Model file for the job. Use its own axes, mm. A direction names the side the tool comes from. Coordinates: 2 decimals unless noted, no trailing zeros. Write each loop counter-clockwise with the first axis right and the second up, starting at its lowest first coordinate (ties: lowest second). Pieces come first, ordered by that corner, then holes. Notation, with made-up numbers: M -23.75,89.5 L -5.75,89.5 A18 cw -5.75,101.5 Z; hole C -23,-14.5 d7. An arc over 180 degrees is marked long. Use CSV: the item, a comma, the result in double quotes. Start each with the question number.
from build123d import *

# Parameters (mm, degrees)
EXTRUDE_1_DEPTH         = 35
CUT_EXTRUDE_1_DEPTH     = 8
CUT_EXTRUDE_2_DEPTH     = 9
EXTRUDE_2_DEPTH         = 6
CUT_EXTRUDE_3_DEPTH     = 3
SKETCH_9_R              = 2.6
CUT_EXTRUDE_4_DEPTH     = 3
CUT_EXTRUDE_5_DEPTH     = 90
SKETCH_11_R             = 5
SKETCH_11_R_2           = 2.6
EXTRUDE_3_DEPTH         = 2
FILLET_1_R              = 5
CUT_EXTRUDE_6_DEPTH     = 2
CUT_EXTRUDE_START       = -31.92392812
CUT_EXTRUDE_7_OUTLINE_W = 4.6
CUT_EXTRUDE_7_OUTLINE_H = 29
CUT_EXTRUDE_7_DEPTH     = 31.92392812
SKETCH_18_W             = 19.8
SKETCH_18_H             = 6.4
CUT_EXTRUDE_8_DEPTH     = 15
SKETCH_19_W             = 19.8
SKETCH_19_H             = 2
CUT_EXTRUDE_9_DEPTH     = 3


# Read off the part's stored shape, not the designer's step: 切除-拉伸7
with BuildPart() as part:
    # 草图1 → 凸台-拉伸1 (new body)
    with BuildSketch(Plane(origin=(0, 0, 0), x_dir=(0, 0, -1), z_dir=(1, 0, 0))):
        Polygon((0, 0), (9, 0), (15.670644845, -8.538036051), (1, -20), (0, -20), align=None)
    extrude(amount=-EXTRUDE_1_DEPTH)

    # 草图5 → 切除-拉伸1 (cut)
    with BuildSketch(Plane.XY):
        Polygon((-27.4, -8.4), (-7.6, -8.4), (-7.6, -2), (-17.5, -2), (-27.4, -2), align=None)
    extrude(amount=-CUT_EXTRUDE_1_DEPTH, mode=Mode.SUBTRACT)

    # 草图6 → 切除-拉伸2 (cut)
    with BuildSketch(Plane(origin=(0, -12.904366819, -10.081996315), x_dir=(1, 0, 0), z_dir=(0, -0.788010753606721, -0.6156614753256595))):
        Polygon((-7.6, 1.307903218), (-7.6, -5.092096782), (-17.5, -5.092096782), (-27.4, -5.092096782), (-27.4, 1.307903218), align=None)
    extrude(amount=-CUT_EXTRUDE_2_DEPTH, mode=Mode.SUBTRACT)

    # 草图7 → 凸台-拉伸2 (add)
    with BuildSketch(Plane(origin=(0, 4.366330768, -5.58864853), x_dir=(-1, 0, 0), z_dir=(0, 0.6156614753256597, -0.7880107536067209))):
        Polygon((0, -5.540953278), (35, -5.540953278), (35, -16.375876547), (35, -36.375876547), (0, -36.375876547), (0, -16.375876547), align=None)
    extrude(amount=EXTRUDE_2_DEPTH)

    # 草图8 → 切除-拉伸3 (cut)
    with BuildSketch(Plane(origin=(0, 8.06029962, -10.316713052), x_dir=(-1, 0, 0), z_dir=(0, 0.6156614753256597, -0.7880107536067209))):
        with BuildLine():
            ThreePointArc((13.158784289, -23.895181856), (15.019305308, -30.717092258), (21.841215711, -28.856571239))
            Line((21.841215711, -28.856571239), (13.158784289, -23.895181856))
        make_face()
        with BuildLine():
            Line((13.158784289, -23.895181856), (21.841215711, -28.856571239))
            ThreePointArc((21.841215711, -28.856571239), (22.332498244, -27.659216223), (22.5, -26.375876547))
            ThreePointArc((22.5, -26.375876547), (18.783339676, -21.543378304), (13.158784289, -23.895181856))
        make_face()
    extrude(amount=-CUT_EXTRUDE_3_DEPTH, mode=Mode.SUBTRACT)

    # 草图9 → 切除-拉伸4 (cut)
    with BuildSketch(Plane(origin=(0, 6.213315194, -7.952680791), x_dir=(-1, 0, 0), z_dir=(0, 0.6156614753256597, -0.7880107536067209))):
        with Locations(Location((17.5, -26.375876547, 0), (0, 0, 90))):
            Circle(SKETCH_9_R)
    extrude(amount=-CUT_EXTRUDE_4_DEPTH, mode=Mode.SUBTRACT)

    # 草图10 → 切除-拉伸5 (cut)
    with BuildSketch(Plane(origin=(0, 0, 0), x_dir=(0, 0, -1), z_dir=(1, 0, 0))):
        Polygon((12.940053768, 3.078307377), (31.92392812, -21.219943746), (32.711938873, -20.604282271), (13.728064522, 3.693968852), align=None)
    extrude(amount=-CUT_EXTRUDE_5_DEPTH, mode=Mode.SUBTRACT)

    # 草图11 → 凸台-拉伸3 (add)
    with BuildSketch(Plane(origin=(0, 7.444638145, -9.528702298), x_dir=(-1, 0, 0), z_dir=(0, 0.6156614753256598, -0.7880107536067208))):
        with Locations((17.5, -26.375876547)):
            Circle(SKETCH_11_R)
        with Locations(Location((17.5, -26.375876547, 0), (0, 0, 90))):
            Circle(SKETCH_11_R_2, mode=Mode.SUBTRACT)
    extrude(amount=-EXTRUDE_3_DEPTH)

    # 圆角1
    fillet_1_edges = [part.edges().sort_by_distance(p)[0] for p in [
        (-17.5, 3.078307377, -12.940053768),
    ]]
    fillet(fillet_1_edges, radius=FILLET_1_R - 0.0001)  # a hair under: the kernel refuses the full size

    # 草图16 → 切除-拉伸6 (cut)
    with BuildSketch(Plane(origin=(0, -12.904366819, -10.081996315), x_dir=(1, 0, 0), z_dir=(0, -0.788010753606721, -0.6156614753256595))):
        Polygon((-27.4, 1.307903218), (-20, 12.313229507), (-15, 12.313229507), (-7.6, 1.307903218), align=None)
    extrude(amount=-CUT_EXTRUDE_6_DEPTH, mode=Mode.SUBTRACT)

    # 切除-拉伸7 outline → 切除-拉伸7 (cut)
    with BuildSketch(Plane.XY.offset(CUT_EXTRUDE_START)):
        with Locations((-32.7, -11.5)):
            Rectangle(CUT_EXTRUDE_7_OUTLINE_W, CUT_EXTRUDE_7_OUTLINE_H)
        with Locations((-2.3, -11.5)):
            Rectangle(CUT_EXTRUDE_7_OUTLINE_W, CUT_EXTRUDE_7_OUTLINE_H)
    extrude(amount=CUT_EXTRUDE_7_DEPTH, mode=Mode.SUBTRACT)

    # 草图18 → 切除-拉伸8 (cut)
    with BuildSketch(Plane.XY):
        with Locations((-17.5, -5.2)):
            Rectangle(SKETCH_18_W, SKETCH_18_H)
    extrude(amount=-CUT_EXTRUDE_8_DEPTH, mode=Mode.SUBTRACT)

    # 草图19 → 切除-拉伸9 (cut)
    with BuildSketch(Plane(origin=(0, -12.904366819, -10.081996315), x_dir=(1, 0, 0), z_dir=(0, -0.788010753606721, -0.6156614753256595))):
        with Locations((-17.5, -6.092096782)):
            Rectangle(SKETCH_19_W, SKETCH_19_H)
    extrude(amount=-CUT_EXTRUDE_9_DEPTH, mode=Mode.SUBTRACT)


solid = part.part
1) Tool access for faces 4 (the face through (-27.4, -6, -8)), 5 (the face through (-17, -2, -7)), 6 (the face through (-17, 0, -4)), 7 (the face through (-9.7, -20, -0.5)), 8 (the face through (-7.27, -15.46, -6.81)): list every direction of +Z, -Z, +X, -X, +Y, -Y with a clear straight run to the whole face (end or side of a thin tool).
2) Two-plate mould, pull along Y, no slides. Class faces 1 (the face through (-18, -5, -15)), 2 (the face through (-25.1, -20, -0.5)), 3 (the face through (-17.64, -10.29, -6.38)): pulls with the +Y half, pulls with the -Y half, needs draft (parallel to the pull), parting line crosses it, or undercut.
3) Band-saw the part on A-A on y = -9. List the corners of the cut face in (x, z), then the cut area to 3 significant figures.
4) Wall check: L1, parallel to Y at x = -17, z = -6; L2, parallel to Z at x = -15.5, y = -10; L3, parallel to X at y = -8.5, z = -6. Give the ranges that are in metal, low to high. Write a range as [from, to].
5) Drop flat-ended pins along their axis: P1, Ø1.1, axis at x = -24.5, z = -0.5, coming from the -Y side; P2, Ø4.5, axis at x = -14.5, z = -6, coming from the -Y side; P3, Ø8, axis at x = -16, y = -6, coming from the -Z side; P4, Ø1.5, axis at y = -15.5, z = -7, coming from the -X side. Give the stop position or say it passes through.
6) Band-saw the part on C-C on z = -10. List the corners of the cut face in (x, y).
Findings below:
1,face 4,"none"
1,face 5,"+Z"
1,face 6,"+Z, +X, -X, +Y"
1,face 7,"+Z, +X, -X, -Y"
1,face 8,"+X, -X, -Y"
2,face 1,"needs draft"
2,face 2,"pulls with the -Y half"
2,face 3,"undercut"
3,outline,"M -30.4,-22.38 L -4.6,-22.38 L -4.6,-16.03 L -30.4,-16.03 Z; M -30.4,-15.08 L -27.4,-15.08 L -27.4,-5.37 L -7.6,-5.37 L -7.6,-15.08 L -4.6,-15.08 L -4.6,0 L -30.4,0 Z"
3,area,"361 mm2"
4,L1,"y = [-13.56, -9.8], [-2, 0]"
4,L2,"z = [-23.16, -16.81], [-6.15, 0]"
4,L3,"x = [-30.4, -27.4], [-7.6, -4.6]"
5,P1,"stops at y = -20"
5,P2,"stops at y = -15.31"
5,P3,"stops at z = -23.16"
5,P4,"stops at x = -30.4"
6,outline,"M -30.4,-12.97 L -27.4,-12.97 L -27.4,-2 L -7.6,-2 L -7.6,-12.97 L -4.6,-12.97 L -4.6,0.61 L -30.4,0.61 Z"
